Autodesk Inventor part; units mm, degrees
ref_plane "YZ Plane" through (0, 0, 0) normal (1, 0, 0) x (0, 1, 0)
ref_plane "XZ Plane" through (0, 0, 0) normal (0, 1, 0) x (-1, 0, 0)
ref_plane "XY Plane" through (0, 0, 0) normal (0, 0, 1) x (1, 0, 0)
sketch "Szkic1" plane through (0, 0, 0) normal (0, 1, 0) x (-1, 0, 0)
  circle A0 centre (0, 0) radius 9.5
  circle A1 centre (0, 0) radius 15
  dimension "d0" = 19
  dimension "d3" = 30
extrude "Wyciągnięcie proste1" add sketch "Szkic1" along normal blind 7
sketch "Szkic2" plane through (0, 7, 0) normal (0, 1, 0) x (1, 0, 0)
  circle A0 centre (0, 0) radius 9.5
  circle A1 centre (0, 0) radius 8.5
  dimension "d4" = 19
  dimension "d5" = 17
extrude "Wyciągnięcie proste2" add sketch "Szkic2" against normal blind 1
chamfer "Faza1" distance 1 distance2 2 1 edges at (15, 0, 0) measured on face at (-14.8058, 4.6667, -2.4062)
properties part number "opona_nosne_dummie" material "Aluminum 6061"
The model under review builds one solid part; all positions refer to its coordinate system, in mm. A direction names the side the tool comes from. Coordinates: 2 decimals unless noted, no trailing zeros. Write each loop counter-clockwise with the first axis right and the second up, starting at its lowest first coordinate (ties: lowest second). Pieces come first, ordered by that corner, then holes. Notation, with made-up numbers: (28.25, 63) -> (78.25, 63) arc R10 cw to (78.25, 76) -> close; hole circle Ø8 at (47, 62). An arc over 180 degrees is marked (long way). One line per item, written item: value. Start each with the question number.
Q1. To check wall thickness, follow probe 1 along Z at (x, y) = (0, 4.4); probe 2 along Z at (x, y) = (0, 6.65); probe 3 along Y at (x, z) = (5.5, 6.75). State the ranges of each line that lie inside material, in increasing order.
Q2. The part is to be moulded in two halves that separate along X. For faces 3 (the face through (-4.38, 2.96, 8.43)), 4 (the face through (14.985, 3.958, -0.66)), 5 (the face through (-1, 0, -10)), say which applies: +X half, -X half, draft (parallel to the pull), parting line (faces both ways), or undercut.
Q3. For faces 1 (the face through (4.57, 6.507, -7.167)), 2 (the face through (-2.2, 6, 8.4)), list the 3-axis set-ups (+Z, -Z, +X, -X, +Y, -Y) from which the entire face can be reached by the end or side of a thin tool; tool diameter is ignored.
Q4. Add section C-C, the plane y = 3.25. Give the boundary of the cut face in (x, z), then the cut area to 3 significant figures.
Q5. Clearance check with flat-ended pins moving along their axes: P1, Ø1.5, axis at x = -9, y = 5.5, coming from the +Z side; P2, Ø4, axis at x = -6.5, z = 2.5, coming from the -Y side. State where each tip first meets the part, or that it passes through.
Q6. Add section B-B, the plane x = 0. Give the boundary of the cut face in (y, z), then the cut area to 3 significant figures.
Q7. Add section A-A, the plane z = 0. Give the boundary of the cut face in (x, y).
Response:
1. probe 1: -15 to -9.5, 9.5 to 15
1. probe 2: -15 to -8.5, 8.5 to 15
1. probe 3: 6 to 7
2. face 3: undercut
2. face 4: parting line
2. face 5: draft
3. face 1: +Y, -Y
3. face 2: -Y
4. outline: circle Ø30 at (0, 0); hole circle Ø19 at (0, 0)
4. area: 423 mm²
5. P1: z = 12.53
5. P2: y = 6
6. outline: (0, -13) -> (1, -15) -> (7, -15) -> (7, -8.5) -> (6, -8.5) -> (6, -9.5) -> (0, -9.5) -> close; (0, 9.5) -> (6, 9.5) -> (6, 8.5) -> (7, 8.5) -> (7, 15) -> (1, 15) -> (0, 13) -> close
6. area: 77.0 mm²
7. outline: (-15, 1) -> (-13, 0) -> (-9.5, 0) -> (-9.5, 6) -> (-8.5, 6) -> (-8.5, 7) -> (-15, 7) -> close; (8.5, 6) -> (9.5, 6) -> (9.5, 0) -> (13, 0) -> (15, 1) -> (15, 7) -> (8.5, 7) -> close
